Read the model definition and answer for the solid it produces. Units are mm, in the model's axes. A direction names the side the tool comes from. Give positions to 0.01 mm unless a question says otherwise; leave off trailing zeros. Order: outer loops, then holes, each group sorted by start corner. A loop starts at its lowest first (then second) coordinate and runs counter-clockwise, first axis right, second up. Notation, with made-up numbers: (-34.75, -4) - (3.25, -4) arc R13 cw to (3.25, 14) - close; hole circle Ø7 at (62.25, 62.25). An arc over 180 degrees is marked (long way). Use a Markdown table: item, result. Add a question column.
1. For a pull along X with two mould halves and no side action, classify faces 1 (the flat face through (-31.115, -1, 12)), 2 (the flat face through (0, 1, 0)), 3 (the flat face through (9, 31, 6.35)), 4 (the flat face through (31.115, 0, 12)) as released by +X, released by -X, zero draft, split by the parting line, or undercut.
2. A cutting plane is placed at B-B on x = -9.5. Determine the outline of the cut face in (y, z), and give its area (3 significant figures).
3. Flat-ended cylindrical pins translate along their axes: P1, Ø5, axis at x = 16, z = 6, coming from the -Y side; P2, Ø0.9, axis at x = 9.5, y = 33, coming from the +Z side; P3, Ø8, axis at x = 0, y = 25, coming from the +Z side. Find the tip coordinate at first contact, or state that the pin passes through.
4. Which of the six approach directions +Z, -Z, +X, -X, +Y, -Y give full straight-line access (tool end or side, diameter ignored) to faces 5 (the flat face through (12, -37.782, 13)), 6 (the flat face through (-27.305, -1, 14)), 7 (the flat face through (18, -37, 7.62))?
5. Consider L1, parallel to Y at x = 7, z = 4.5; L2, parallel to Y at x = -19, z = 10.25; L3, parallel to X at y = -22.5, z = 7.5 (3 decimals). Determine where each line is inside the solid, lowest interval first.
6. A cutting plane is placed at C-C on y = -5. Determine the outline of the cut face in (x, z) (3 decimals), and give its area (3 significant figures).
7. A cutting plane is placed at D-D on z = 21.5. Determine the outline of the cut face in (x, y) (1 decimal), and give its area (3 significant figures).
8. A cutting plane is placed at A-A on z = 15.75. Determine the outline of the cut face in (x, y) (1 decimal), and give its area (3 significant figures).
```python
from build123d import *

# Parameters (mm, degrees)
F0_W      = 62.23
F0_H      = 79.375
F1_DEPTH  = 24.13
F2_T      = -3.81
F4_R      = 2.54
F5_DEPTH  = 2.54
F7_R      = 1.524
F8_DEPTH  = 7.62
F9_W      = 12.954
F9_H      = 10.922
F9_W_2    = 9.144
F9_H_2    = 11.176
F10_DEPTH = 3.81
F11_W     = 31.115
F11_H     = 24.13
F12_DEPTH = 1.905
F13_SIZE  = 0.889


with BuildPart() as f1:
    # F0 (on Top) → F1 (new body)
    with BuildSketch(Plane.XY):
        Rectangle(F0_W, F0_H)
    extrude(amount=F1_DEPTH)

    # F2
    f2_openings = [f1.faces().sort_by_distance(p)[0] for p in [
        (0, 0, 24.13),
    ]]
    offset(amount=F2_T, openings=f2_openings)

    # F4 (on face) → F5 (join)
    with BuildSketch(Plane.XY.offset(3.81)):
        with Locations((9.017, 32.7025)):
            Circle(F4_R)
        with Locations((-18.923, 32.7025)):
            Circle(F4_R)
        with Locations((-24.003, -19.3675)):
            Circle(F4_R)
        with Locations((24.13, -18.0975)):
            Circle(F4_R)
    extrude(amount=F5_DEPTH)

    # F7 (on offset) → F8 (join)
    with BuildSketch(Plane.XY.offset(6.35)):
        with Locations((9.017, 32.7025)):
            Circle(F7_R)
        with Locations((-18.923, 32.7025)):
            Circle(F7_R)
        with Locations((-24.003, -19.3675)):
            Circle(F7_R)
        with Locations((24.13, -18.0975)):
            Circle(F7_R)
    extrude(amount=F8_DEPTH)

    # F9 (on face) → F10 (cut, through all)
    with BuildSketch(Plane.XZ.offset(39.6875)):
        with Locations((-10.668, 12.827)):
            Rectangle(F9_W, F9_H)
        with Locations((18.415, 13.208)):
            Rectangle(F9_W_2, F9_H_2)
    extrude(amount=-F10_DEPTH, mode=Mode.SUBTRACT)

    # F11 (on face) → F12 (cut)
    with BuildSketch(Plane.XZ.offset(39.6875)):
        with Locations((15.5575, 12.065)):
            Rectangle(F11_W, F11_H)
    extrude(amount=-F12_DEPTH, mode=Mode.SUBTRACT)

    # F13
    f13_edges = [f1.edges().sort_by_distance(p)[0] for p in [
        (-15.5575, -39.6875, 24.13),
        (-31.115, 0, 24.13),
        (0, 39.6875, 24.13),
        (31.115, 39.6875, 12.065),
        (31.115, 0.9525, 24.13),
        (31.115, -37.7825, 12.065),
        (31.115, 0.9525, 0),
        (15.5575, -37.7825, 0),
        (0, -39.6875, 12.065),
        (-15.5575, -39.6875, 0),
        (-31.115, -39.6875, 12.065),
        (-31.115, 39.6875, 12.065),
        (-31.115, 0, 0),
        (0, 39.6875, 0),
    ]]
    chamfer(f13_edges, length=F13_SIZE)


solid = f1.part
```
Output values:
| question | item | result |
|---|---|---|
| 1 | face 1 | released by -X |
| 1 | face 2 | zero draft |
| 1 | face 3 | undercut |
| 1 | face 4 | released by +X |
| 2 | outline | (-39.69, 0.89) - (-38.8, 0) - (38.8, 0) - (39.69, 0.89) - (39.69, 23.24) - (38.8, 24.13) - (35.88, 24.13) - (35.88, 3.81) - (-35.88, 3.81) - (-35.88, 7.37) - (-39.69, 7.37) - close; (-39.69, 18.29) - (-35.88, 18.29) - (-35.88, 24.13) - (-38.8, 24.13) - (-39.69, 23.24) - close |
| 2 | area | 414 mm² |
| 3 | P1 | y = -37.78 |
| 3 | P2 | z = 13.97 |
| 3 | P3 | z = 3.81 |
| 4 | face 5 | +Z, -Z, +X, -Y |
| 4 | face 6 | +Z |
| 4 | face 7 | -Y |
| 5 | L1 | -37.78 to -35.88, 31.16 to 34.25, 35.88 to 39.69 |
| 5 | L2 | -39.69 to -35.88, 31.18 to 34.22, 35.88 to 39.69 |
| 5 | L3 | -31.115 to -27.305, 27.305 to 31.115 |
| 6 | outline | (-31.115, 0.889) - (-30.226, 0) - (30.226, 0) - (31.115, 0.889) - (31.115, 23.241) - (30.226, 24.13) - (27.305, 24.13) - (27.305, 3.81) - (-27.305, 3.81) - (-27.305, 24.13) - (-30.226, 24.13) - (-31.115, 23.241) - close |
| 6 | area | 390 mm² |
| 7 | outline | (-31.1, -38.8) - (-30.2, -39.7) - (-0.9, -39.7) - (0, -38.8) - (0, -37.8) - (30.2, -37.8) - (31.1, -36.9) - (31.1, 38.8) - (30.2, 39.7) - (-30.2, 39.7) - (-31.1, 38.8) - close; hole (-27.3, -35.9) - (27.3, -35.9) - (27.3, 35.9) - (-27.3, 35.9) - close |
| 7 | area | 960 mm² |
| 8 | outline | (-31.1, -38.8) - (-30.2, -39.7) - (-17.1, -39.7) - (-17.1, -35.9) - (-27.3, -35.9) - (-27.3, 35.9) - (27.3, 35.9) - (27.3, -35.9) - (23, -35.9) - (23, -37.8) - (30.2, -37.8) - (31.1, -36.9) - (31.1, 38.8) - (30.2, 39.7) - (-30.2, 39.7) - (-31.1, 38.8) - close; (-4.2, -39.7) - (-0.9, -39.7) - (0, -38.8) - (0, -37.8) - (13.8, -37.8) - (13.8, -35.9) - (-4.2, -35.9) - close |
| 8 | area | 893 mm² |
